Source: three-view drawing plus pictorial views. Frame: mm from the lowest corner of the part. Coordinates: 2 decimals unless noted, no trailing zeros. Loops run counter-clockwise (first coordinate to the right, second up) from the corner with the lowest first, then second, coordinate; pieces in that order, holes last. Notation, with made-up numbers: (39, 45.5) - (64, 45.5) arc R27 cw to (64, 67.5) - close; hole circle Ø9 at (10, 51.5). An arc over 180 degrees is marked (long way). Return JSON: item names as keys, results as strings.
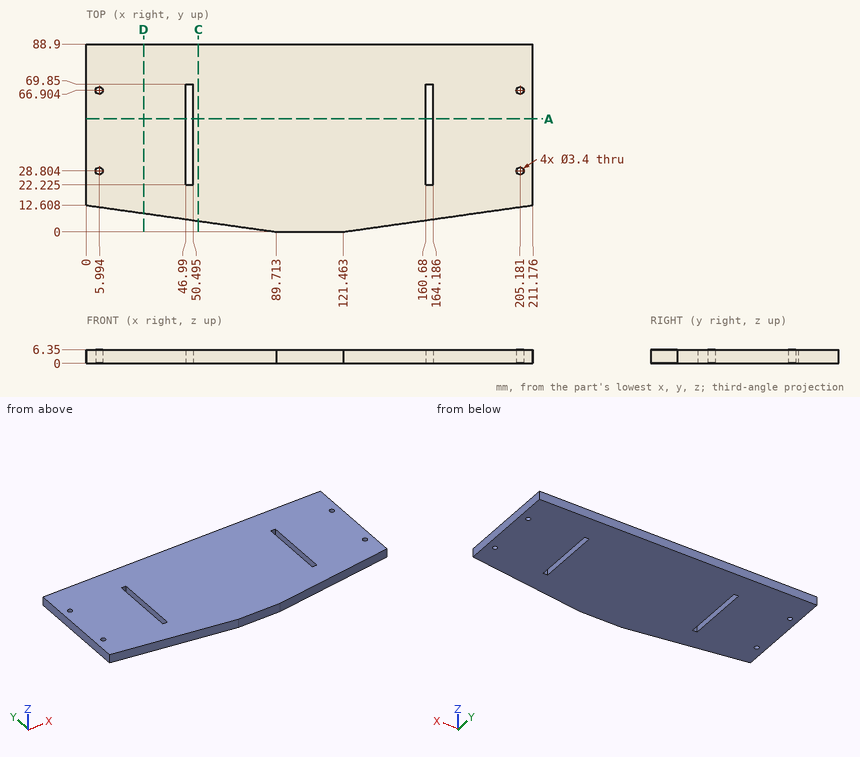
Item 1: Section query D-D, the plane x = 27. Return loops of the section in (y, z).
Worked out:
{"outline": "(8.81, 0) - (88.9, 0) - (88.9, 6.35) - (8.81, 6.35) - close"}
Item 2: Section query A-A, the plane y = 53.5. Count the separate pieces of the cut face and the enclosed holes in it, and give its area (3 significant figures).
Worked out:
{"separate pieces": "3", "enclosed holes": "0", "area": "1,300 mm^2"}
Item 3: Section query C-C, the plane x = 53. Return loops of the section in (y, z).
Worked out:
{"outline": "(5.16, 0) - (88.9, 0) - (88.9, 6.35) - (5.16, 6.35) - close"}
Item 4: Ray query, probe 1 along X at (y, z) = (31.5, 2.25) (1 decimal); probe 2 along X at (y, z) = (66.5, 3) (1 decimal); probe 3 along X at (y, z) = (29, 6) (1 decimal). Return the intervals inside material, ascending. Write a range as from..to.
Worked out:
{"probe 1": "0..47, 50.5..160.7, 164.2..211.2", "probe 2": "0..4.3, 7.6..47, 50.5..160.7, 164.2..203.5, 206.8..211.2", "probe 3": "0..4.3, 7.7..47, 50.5..160.7, 164.2..203.5, 206.9..211.2"}
Item 5: First-contact query: pin 1 Ø2 at (x, y) = (205.18, 28.8) entering from +Z; pin 2 Ø5.5 at (x, y) = (205.18, 66.9) entering from +Z; pin 3 Ø3 at (x, z) = (163.5, 4) entering from -Y; pin 4 Ø3 at (x, z) = (49, 4) entering from -Y. Flat tips, straight axial feed; report the tip coordinate or a pass-through.
Worked out:
{"pin 1": "through", "pin 2": "z = 6.35", "pin 3": "y = 5.7", "pin 4": "y = 5.51"}
